Part model, mm, in its own coordinate system. A direction names the side the tool comes from. Round coordinates to 2 decimals unless told otherwise and drop trailing zeros. Loops run counter-clockwise (first coordinate to the right, second up) from the corner with the lowest first, then second, coordinate; pieces in that order, holes last.
1) Band-saw the part on B-B, the plane y = -0.5. Write the cut outline in (x, z), then the cut area to 3 significant figures.
2) Band-saw the part on A-A, the plane x = 0. Write the cut outline in (y, z), then the cut area to 3 significant figures.
3) Mould opens along Z. For faces 4 (the flat face through (0, 0, 0)), 5 (the flat face through (0, 0, 4.5)), 6 (the flat face through (1, 0, 3)) say: +Z half, -Z half, draft (parallel to the pull), parting line (faces both ways), or undercut.
4) Probe line 1 (Z direction, x = 5.5, y = 2.25); line 2 (X direction, y = -1.5, z = 2.65); line 3 (Y direction, x = 0.25, z = 3.25). List the from-to ranges inside material, lowest first.
5) Band-saw the part on C-C, the plane z = 2.2. Write the cut outline in (x, y), then the cut area to 3 significant figures.
6) 3-axis set-ups, long thin cutter, end or side, ignore diameter. For faces 1 (the cylindrical face through (0, 3, 3)), 2 (the flat face through (-1, 0, 3)), 3 (the cylindrical face through (0, -3, 3)): which of +Z, -Z, +X, -X, +Y, -Y reach the whole face in a straight line?
7) Band-saw the part on D-D, the plane x = 4.25. Write the cut outline in (y, z), then the cut area to 3 significant figures.
8) Drop flat-ended pins along their axis: P1, Ø0.9, axis at y = -1, z = 3.5, coming from the -X side; P2, Ø2, axis at x = 3.5, z = 3.5, coming from the -Y side; P3, Ø2, axis at y = -2, z = 3, coming from the +X side. Give the stop position or say it passes through.
from build123d import *

# Parameters (mm, degrees)
F0_W     = 17
F0_H     = 7
F1_DEPTH = 1.5
F2_W     = 2
F2_H     = 4
F3_DEPTH = 3
F4_R     = 1


with BuildPart() as f1:
    # F0 (on Top) → F1 (new body)
    with BuildSketch(Plane.XY):
        Rectangle(F0_W, F0_H)
    extrude(amount=F1_DEPTH)

    # F2 (on face) → F3 (join)
    with BuildSketch(Plane.XY.offset(1.5)):
        with BuildLine():
            ThreePointArc((-1, -2), (0, -3), (1, -2))
            Line((1, -2), (-1, -2))
        make_face()
        Rectangle(F2_W, F2_H)
        with BuildLine():
            Line((-1, 2), (1, 2))
            ThreePointArc((1, 2), (0, 3), (-1, 2))
        make_face()
    extrude(amount=F3_DEPTH)

    # F4
    f4_edges = [f1.edges().sort_by_distance(p)[0] for p in [
        (-8.5, 3.5, 0.75),
        (-8.5, -3.5, 0.75),
        (8.5, 3.5, 0.75),
        (8.5, -3.5, 0.75),
    ]]
    fillet(f4_edges, radius=F4_R)


solid = f1.part
Reported:
1. outline: (-8.5, 0) - (8.5, 0) - (8.5, 1.5) - (1, 1.5) - (1, 4.5) - (-1, 4.5) - (-1, 1.5) - (-8.5, 1.5) - close
1. area: 31.5 mm2
2. outline: (-3.5, 0) - (3.5, 0) - (3.5, 1.5) - (3, 1.5) - (3, 4.5) - (-3, 4.5) - (-3, 1.5) - (-3.5, 1.5) - close
2. area: 28.5 mm2
3. face 4: -Z half
3. face 5: +Z half
3. face 6: draft
4. line 1: z = 0 to 1.5
4. line 2: x = -1 to 1
4. line 3: y = -2.97 to 2.97
5. outline: (-1, -2) arc R1 ccw to (1, -2) - (1, 2) arc R1 ccw to (-1, 2) - close
5. area: 11.1 mm2
6. face 1: +Z, +Y
6. face 2: +Z, -X, +Y, -Y
6. face 3: +Z, -Y
7. outline: (-3.5, 0) - (3.5, 0) - (3.5, 1.5) - (-3.5, 1.5) - close
7. area: 10.5 mm2
8. P1: stops at x = -1
8. P2: passes through
8. P3: stops at x = 1
